Source: CAD feature listing. Evaluate the final solid. Frame: model axes, mm. Face numbers are marked on the shaded views. A direction names the side the tool comes from. Give positions to 0.01 mm unless a question says otherwise; leave off trailing zeros. Write each loop counter-clockwise with the first axis right and the second up, starting at its lowest first coordinate (ties: lowest second). Pieces come first, ordered by that corner, then holes.
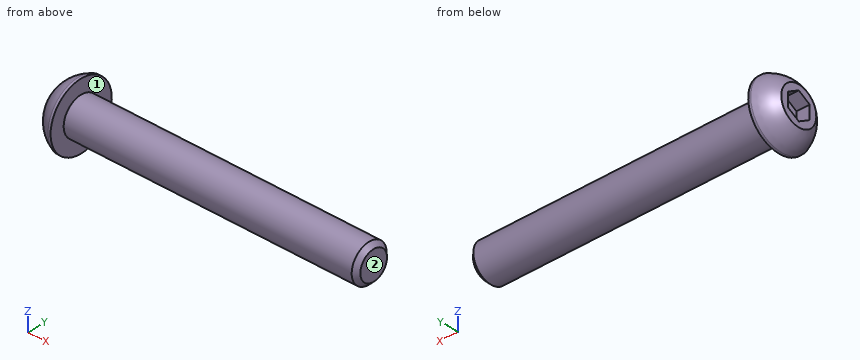
```python
from build123d import *

# Parameters (mm, degrees)
SKETCH2_R           = 3.175
BOSS_EXTRUDE1_DEPTH = 49.149
CUT_EXTRUDE1_DEPTH  = 2.2225
CHAMFER1_SIZE       = 0.75565


with BuildPart() as part:
    # Sketch1 → Revolve1 (revolve)
    with BuildSketch(Plane.XY, mode=Mode.PRIVATE) as revolve1_sk:
        with BuildLine():
            Line((-3.3528, 3.175), (-3.3528, 0))
            Line((-3.3528, 0), (0, 0))
            Line((0, 0), (0, 5.5499))
            Line((0, 5.5499), (-0.4318, 5.5499))
            ThreePointArc((-0.4318, 5.5499), (-2.086170702, 4.600900596), (-3.3528, 3.175))
        make_face()
    revolve(revolve1_sk.sketch.rotate(Axis((-3.3528, 0, 0), (1, 0, 0)), 270), axis=Axis((-3.3528, 0, 0), (1, 0, 0)))

    # Sketch2 → Boss-Extrude1 (add)
    with BuildSketch(Plane(origin=(0, 0, 0), x_dir=(0, 0, -1), z_dir=(1, 0, 0))):
        with Locations(Location((0, 0, 0), (0, 0, 180))):
            Circle(SKETCH2_R)
    extrude(amount=BOSS_EXTRUDE1_DEPTH)

    # Sketch3 → Cut-Extrude1 (cut)
    with BuildSketch(Plane.ZY.offset(3.3528)):
        Polygon((2.291358881, 0), (1.14567944, 1.984375), (-1.14567944, 1.984375), (-2.291358881, 0), (-1.14567944, -1.984375), (1.14567944, -1.984375), align=None)
    extrude(amount=-CUT_EXTRUDE1_DEPTH, mode=Mode.SUBTRACT)

    # Chamfer1
    chamfer1_edges = [part.edges().sort_by_distance(p)[0] for p in [
        (49.149, 0, -3.175),
    ]]
    chamfer(chamfer1_edges, length=CHAMFER1_SIZE)


solid = part.part
```
1. Line query: probe 1 along Y at (x, z) = (1, 0) (3 decimals); probe 2 along Z at (x, y) = (33, -0.25); probe 3 along X at (y, z) = (0.75, -0.5). Output: solid intervals per line, ascending.
2. Section query A-A (x = 2). Return loops of the section in (y, z) (3 decimals).
3. Access query for the marked faces 1 and 2. Directions: +Z, -Z, +X, -X, +Y, -Y. A direction counts if a zero-diameter tool reaches every point of the face in a straight line with its end or side. Return the directions, or none.
4. Pin query (flat end, axial travel): P1, Ø5, axis at x = 11, z = -1, coming from the -Y side (3 decimals); P2, Ø2.5, axis at x = -2, z = 0.5, coming from the +Y side; P3, Ø2, axis at x = 33.5, z = 1, coming from the +Y side (3 decimals); P4, Ø4.5, axis at y = 0.5, z = 0, coming from the -X side. Return the tip coordinate at first contact, or that it passes through.
The answers:
1. probe 1: y = -3.175 to 3.175
1. probe 2: z = -3.17 to 3.17
1. probe 3: x = -1.13 to 49.15
2. outline: circle Ø6.35 at (0, 0)
3. face 1: +X
3. face 2: +Z, -Z, +X, +Y, -Y
4. P1: stops at y = -3.175
4. P2: stops at y = 5.4
4. P3: stops at y = 3.175
4. P4: stops at x = -3.35
